For this review, take the finished solid that the model builds, in its own axes (mm). A direction names the side the tool comes from. Give positions to 0.01 mm unless a question says otherwise; leave off trailing zeros. Write each loop counter-clockwise with the first axis right and the second up, starting at its lowest first coordinate (ties: lowest second). Pieces come first, ordered by that corner, then holes. Notation, with made-up numbers: (-18.75, 63) -> (35.25, 63) arc R25 ccw to (35.25, 78) -> close; hole circle Ø5 at (-12, -3.5). An arc over 180 degrees is marked (long way). Write item = value, one per line.
```python
from build123d import *

# Parameters (mm, degrees)
F0_W     = 100
F0_H     = 40
F1_DEPTH = 1
F2_W     = 100
F2_H     = 40
F2_W_2   = 96
F2_H_2   = 36
F3_DEPTH = 20
F4_W     = 3
F4_H     = 2
F5_DEPTH = 25
F6_W     = 19
F6_H     = 13
F7_DEPTH = 25
F8_R     = 1


with BuildPart() as f1:
    # F0 (on Top) → F1 (new body)
    with BuildSketch(Plane.XY):
        with Locations((50, 20)):
            Rectangle(F0_W, F0_H)
    extrude(amount=F1_DEPTH)

    # F2 (on face) → F3 (join)
    with BuildSketch(Plane.XY.offset(1)):
        with Locations((50, 20)):
            Rectangle(F2_W, F2_H)
        with Locations((50, 20)):
            Rectangle(F2_W_2, F2_H_2, mode=Mode.SUBTRACT)
    extrude(amount=F3_DEPTH)

    # F4 (on face) → F5 (cut)
    with BuildSketch(Plane.YZ.offset(100)):
        with Locations((28.5, 2)):
            Rectangle(F4_W, F4_H)
    extrude(amount=-F5_DEPTH, mode=Mode.SUBTRACT)

    # F6 (on face) → F7 (cut)
    with BuildSketch(Plane.XZ):
        with Locations((80.5, 10.5)):
            Rectangle(F6_W, F6_H)
    extrude(amount=-F7_DEPTH, mode=Mode.SUBTRACT)

    # F8
    f8_edges = [f1.edges().sort_by_distance(p)[0] for p in [
        (0, 0, 10.5),
        (100, 0, 10.5),
        (100, 40, 10.5),
        (0, 40, 10.5),
    ]]
    fillet(f8_edges, radius=F8_R)


solid = f1.part
```
(1) Tool access review of faces 1 (the face through (90, 1, 10)), 2 (the face through (49, 38, 11)), 3 (the face through (99, 28, 3)): name each direction out of +Z, -Z, +X, -X, +Y, -Y from which nothing blocks a thin tool from reaching the whole face with its end or side.
Answers below:
face_1 = -Y
face_2 = +Z
face_3 = +X
(2) Take a section at D-D (y = 24). Write out the cut boundary in (x, z), plus the area to 3 significant figures.
Answers below:
outline = (0, 0) -> (100, 0) -> (100, 21) -> (98, 21) -> (98, 1) -> (2, 1) -> (2, 21) -> (0, 21) -> close
area = 180 mm^2
(3) Take a section at A-A (y = 29). Write out the cut boundary in (x, z), plus the area to 3 significant figures.
Answers below:
outline = (0, 0) -> (100, 0) -> (100, 1) -> (2, 1) -> (2, 21) -> (0, 21) -> close; (98, 3) -> (100, 3) -> (100, 21) -> (98, 21) -> close
area = 176 mm^2
(4) To check wall thickness, follow probe 1 along X at (y, z) = (22.5, 15.75); probe 2 along Y at (x, z) = (32, 3.75); probe 3 along Z at (x, y) = (77.5, 12). State the ranges of each line that lie inside material, in increasing order.
Answers below:
probe_1 = 0 to 2, 98 to 100
probe_2 = 0 to 2, 38 to 40
probe_3 = 0 to 1
(5) Take a section at C-C (z = 16). Write out the cut boundary in (x, y), plus the area to 3 significant figures.
Answers below:
outline = (0, 1) arc R1 ccw to (1, 0) -> (71, 0) -> (71, 2) -> (2, 2) -> (2, 38) -> (98, 38) -> (98, 2) -> (90, 2) -> (90, 0) -> (99, 0) arc R1 ccw to (100, 1) -> (100, 39) arc R1 ccw to (99, 40) -> (1, 40) arc R1 ccw to (0, 39) -> close
area = 505 mm^2
(6) For pin 1 (12 mm diameter, centred on x = 18.5, y = 19, fed in from +Z), flat-tipped, find the tip position at first contact; note if it passes through.
Answers below:
pin_1 = 1
(7) The part is to be moulded in two halves that separate along X. For faces 4 (the face through (0, 20, 10)), 5 (the face through (49, 40, 10)), 6 (the face through (80, 1, 4)), say which applies: released by +X, released by -X, zero draft, split by the parting line, or undercut.
Answers below:
face_4 = released by -X
face_5 = zero draft
face_6 = undercut
(8) Take a section at B-B (x = 88.5). Write out the cut boundary in (y, z).
Answers below:
outline = (0, 0) -> (40, 0) -> (40, 21) -> (38, 21) -> (38, 1) -> (2, 1) -> (2, 4) -> (0, 4) -> close; (0, 17) -> (2, 17) -> (2, 21) -> (0, 21) -> close
